The model under review builds one solid part; all positions refer to its coordinate system, in mm. Face numbers are marked on the shaded views. Give positions to 0.01 mm unless a question says otherwise; leave off trailing zeros. Loops run counter-clockwise (first coordinate to the right, second up) from the corner with the lowest first, then second, coordinate; pieces in that order, holes last. Notation, with made-up numbers: M 45,69 L 69,69 A12 cw 69,76 Z; hole C 70.5,19 d10. An arc over 180 degrees is marked long. One line per item, written item: value. Start each with the question number.
Q1. To check wall thickness, follow line 1 along Z through (x, y) = (0.25, 15); line 2 along X through (y, z) = (15.3, 23.5); line 3 along Y through (x, z) = (0.35, 21.75). State the ranges of each line that lie inside material, in increasing order. Write a range as from..to.
Q2. We need section A-A on x = 0. Write out the cut boundary in (y, z), plus the area to 3 significant figures.
Q3. We need section C-C on z = 23.25. Write out the cut boundary in (x, y), plus the area to 3 significant figures.
Q4. For pin 1 (1.5 mm diameter, centred on x = -0.5, y = 16.5, fed in from -Z); pin 2 (2 mm diameter, centred on y = 17, z = 25.5, fed in from -X); pin 3 (1 mm diameter, centred on x = 0, z = 21.5, fed in from +Y), all flat-tipped, find the tip position at first contact; note any pin that passes through.
Q5. Mouldability with a two-part tool opening along Y and no side actions: class the marked faces 1, 2 and 3 as released by +Y, released by -Y, zero draft, split by the parting line, or undercut.
Q6. We need section D-D on x = 1.05. Write out the cut boundary in (y, z), plus the area to 3 significant figures.
Q7. We need section B-B on y = 15.24. Write out the cut boundary in (x, z).
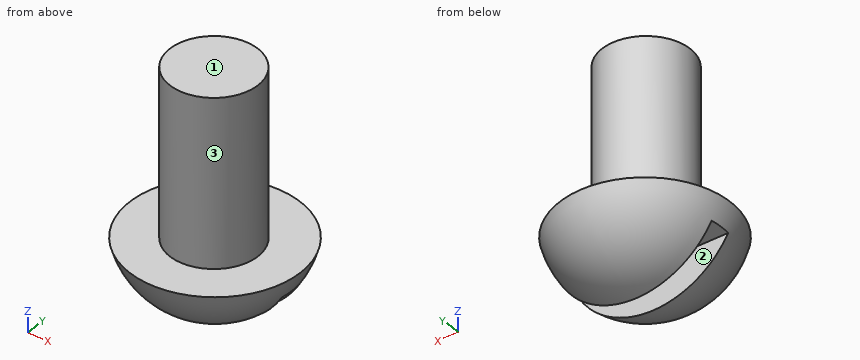
```python
from build123d import *

# Parameters (mm, degrees)
SKETCH2_R           = 1.2573
BOSS_EXTRUDE1_DEPTH = 4.7752
CUT_EXTRUDE1_DEPTH  = 3.434750981


with BuildPart() as part:
    # Sketch1 → Base-Revolve (revolve)
    with BuildSketch(Plane(origin=(0, 0, 0), x_dir=(0, 0, -1), z_dir=(1, 0, 0))):
        with BuildLine():
            Line((-22.86, 15.282157927), (-20.97405, 15.282157927))
            ThreePointArc((-20.97405, 15.282157927), (-21.500684149, 16.822029654), (-22.86, 17.716908908))
            Line((-22.86, 17.716908908), (-22.86, 15.282157927))
        make_face()
    revolve(axis=Axis((0, 15.282157927, 28.59405), (0, 0, -1)))

    # Sketch2 → Boss-Extrude1 (add)
    with BuildSketch(Plane.XY.offset(22.86)):
        with Locations((0, 15.24)):
            Circle(SKETCH2_R)
    extrude(amount=BOSS_EXTRUDE1_DEPTH)

    # Sketch4 → Cut-Extrude1 (cut, through all)
    with BuildSketch(Plane(origin=(0, 0, 0), x_dir=(0, 0, -1), z_dir=(1, 0, 0))):
        with BuildLine():
            Line((-22.251072657, 14.967832927), (-20.993772657, 14.967832927))
            ThreePointArc((-20.993772657, 14.967832927), (-20.97405, 15.282157927), (-20.993772657, 15.596482927))
            Line((-20.993772657, 15.596482927), (-22.251072657, 15.596482927))
            Line((-22.251072657, 15.596482927), (-22.251072657, 14.967832927))
        make_face()
    cut_extrude1 = extrude(amount=-CUT_EXTRUDE1_DEPTH, mode=Mode.SUBTRACT)

    # Mirror1: Cut-Extrude1 across plane
    add(cut_extrude1.mirror(Plane(origin=(0, 15.282157927, 23.48865), x_dir=(0, 0, 1), z_dir=(1, 0, 0))), mode=Mode.SUBTRACT)


solid = part.part
```
Solved:
1. line 1: 22.25..27.64
1. line 2: -1.26..1.26
1. line 3: 13.5..14.97, 15.6..17.06
2. outline: M 12.85,22.86 A2.51 ccw 14.97,20.99 L 14.97,22.25 L 15.6,22.25 L 15.6,20.99 A2.51 ccw 17.72,22.86 L 16.5,22.86 L 16.5,27.64 L 13.98,27.64 L 13.98,22.86 Z
2. area: 18.0 mm2
3. outline: C 0,15.24 d2.51
3. area: 4.97 mm2
4. pin 1: z = 21.04
4. pin 2: x = -1
4. pin 3: y = 17.31
5. face 1: zero draft
5. face 2: undercut
5. face 3: split by the parting line
6. outline: M 13.09,22.86 A2.28 ccw 14.97,21.23 L 14.97,22.25 L 15.6,22.25 L 15.6,21.23 A2.28 ccw 17.48,22.86 L 15.93,22.86 L 15.93,27.64 L 14.55,27.64 L 14.55,22.86 Z
6. area: 11.3 mm2
7. outline: M -2.43,22.86 A2.51 ccw -2.19,22.25 L 2.19,22.25 A2.51 ccw 2.43,22.86 L 1.26,22.86 L 1.26,27.64 L -1.26,27.64 L -1.26,22.86 Z
